```python
from build123d import *

# Parameters (mm, degrees)
SKETCH_1_W          = 65
SKETCH_1_H          = 45
EXTRUDE_1_DEPTH     = 25
SKETCH_2_R          = 1.5
CUT_EXTRUDE_1_DEPTH = 10


with BuildPart() as part:
    # Эскиз1 → Бобышка-Вытянуть1 (new body)
    with BuildSketch(Plane(origin=(0, 0, 0), x_dir=(1, 0, 0), z_dir=(0, 1, 0))):
        Rectangle(SKETCH_1_W, SKETCH_1_H)
    extrude(amount=EXTRUDE_1_DEPTH)

    # Эскиз2 → Вырез-Вытянуть1 (cut)
    with BuildSketch(Plane.XZ):
        with Locations(Location((-29.5, 13.5, 0), (0, 0, 270))):
            Circle(SKETCH_2_R)
        with Locations(Location((29.5, 13.5, 0), (0, 0, 270))):
            Circle(SKETCH_2_R)
        with Locations(Location((-29.5, -13.5, 0), (0, 0, 270))):
            Circle(SKETCH_2_R)
        with Locations(Location((29.5, -13.5, 0), (0, 0, 270))):
            Circle(SKETCH_2_R)
    extrude(amount=-CUT_EXTRUDE_1_DEPTH, mode=Mode.SUBTRACT)


solid = part.part
```
Model file for the job. Use its own axes, mm. A direction names the side the tool comes from. Coordinates: 2 decimals unless noted, no trailing zeros. Order: outer loops, then holes, each group sorted by start corner. A loop starts at its lowest first (then second) coordinate and runs counter-clockwise, first axis right, second up. Notation, with made-up numbers: (16, 2) - (36, 2) arc R19 ccw to (36, 38) - close; hole circle Ø6 at (33, 61.25). An arc over 180 degrees is marked (long way). Return JSON: item names as keys, results as strings. Group by question number.
1) Probe line 1 (X direction, y = 9.75, z = -13.5). List the from-to ranges inside material, lowest first. Write a range as from..to.
2) Saw through at A-A, the plane z = 13.5. Write the cut outline in (x, y).
3) Tool access for faces 1 (the flat face through (-32.5, 12, 0)), 2 (the cylindrical face through (-28.013, 4.93, 13.695)): list every direction of +Z, -Z, +X, -X, +Y, -Y with a clear straight run to the whole face (end or side of a thin tool).
4) Saw through at B-B, the plane x = -29.5. Write the cut outline in (y, z), plus the area to 4 significant figures.
5) Flat gauge pin, fed straight in: P1, Ø0.9, axis at x = -29, z = 14, coming from the -Y side. Where does the tip first touch, or does it go through?
6) Mould opens along X. For faces 3 (the cylindrical face through (-28.013, 4.93, -13.305)), 4 (the flat face through (0, 0, 0)), 5 (the flat face through (32.5, 12, 0)) say: released by +X, released by -X, zero draft, split by the parting line, or undercut.
Values found:
{
 "1": {"line 1": "x = -32.5..-31, -28..28, 31..32.5"},
 "2": {"outline": "(-32.5, 0) - (-31, 0) - (-31, 10) - (-28, 10) - (-28, 0) - (28, 0) - (28, 10) - (31, 10) - (31, 0) - (32.5, 0) - (32.5, 25) - (-32.5, 25) - close"},
 "3": {"face 1": "+Z, -Z, -X, +Y, -Y", "face 2": "-Y"},
 "4": {"outline": "(0, -22.5) - (25, -22.5) - (25, 22.5) - (0, 22.5) - (0, 15) - (10, 15) - (10, 12) - (0, 12) - (0, -12) - (10, -12) - (10, -15) - (0, -15) - close", "area": "1,065 mm²"},
 "5": {"P1": "stops at y = 10"},
 "6": {"face 3": "undercut", "face 4": "zero draft", "face 5": "released by +X"}
}
